Part model, mm, in its own coordinate system. Face numbers are marked on the shaded views. A direction names the side the tool comes from. Round coordinates to 2 decimals unless told otherwise and drop trailing zeros. Write each loop counter-clockwise with the first axis right and the second up, starting at its lowest first coordinate (ties: lowest second). Pieces come first, ordered by that corner, then holes.
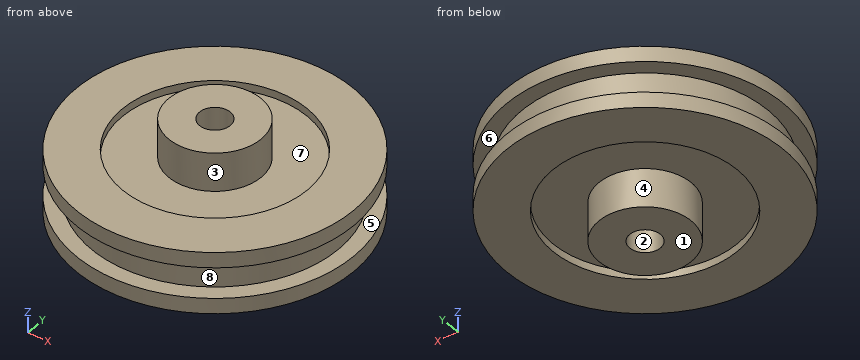
```python
from build123d import *

# Parameters (mm, degrees)
F0_R      = 9
F1_DEPTH  = 4
F2_R      = 6
F3_DEPTH  = 0.5
F4_R      = 6
F5_DEPTH  = 0.5
F6_R      = 3
F7_DEPTH  = 2.5
F8_R      = 3
F9_DEPTH  = 2.5
F10_R     = 1
F11_DEPTH = 25
F13_R     = 15.851527
F13_R_2   = 8
F14_DEPTH = 2


with BuildPart() as f1:
    # F0 (on Top) → F1 (new body)
    with BuildSketch(Plane.XY):
        Circle(F0_R)
    extrude(amount=F1_DEPTH)

    # F2 (on face) → F3 (cut)
    with BuildSketch(Plane(origin=(0, 0, 0), x_dir=(1, 0, 0), z_dir=(0, 0, -1))):
        Circle(F2_R)
    extrude(amount=-F3_DEPTH, mode=Mode.SUBTRACT)

    # F4 (on face) → F5 (cut)
    with BuildSketch(Plane.XY.offset(4)):
        Circle(F4_R)
    extrude(amount=-F5_DEPTH, mode=Mode.SUBTRACT)

    # F6 (on face) → F7 (join)
    with BuildSketch(Plane(origin=(0, 0, 0.5), x_dir=(1, 0, 0), z_dir=(0, 0, -1))):
        Circle(F6_R)
    extrude(amount=F7_DEPTH)

    # F8 (on face) → F9 (join)
    with BuildSketch(Plane.XY.offset(3.5)):
        Circle(F8_R)
    extrude(amount=F9_DEPTH)

    # F10 (on face) → F11 (cut)
    with BuildSketch(Plane.XY.offset(6)):
        Circle(F10_R)
    extrude(amount=-F11_DEPTH, mode=Mode.SUBTRACT)

    # F13 (on offset) → F14 (cut)
    with BuildSketch(Plane.XY.offset(1)):
        Circle(F13_R)
        Circle(F13_R_2, mode=Mode.SUBTRACT)
    extrude(amount=F14_DEPTH, mode=Mode.SUBTRACT)


solid = f1.part
```
Q1. Cut at D-D on y = 4.75. Write the cut outline in (x, z).
Values follow:
outline: (-7.64, 0) - (-3.67, 0) - (-3.67, 0.5) - (3.67, 0.5) - (3.67, 0) - (7.64, 0) - (7.64, 1) - (6.44, 1) - (6.44, 3) - (7.64, 3) - (7.64, 4) - (3.67, 4) - (3.67, 3.5) - (-3.67, 3.5) - (-3.67, 4) - (-7.64, 4) - (-7.64, 3) - (-6.44, 3) - (-6.44, 1) - (-7.64, 1) - close
Q2. Which spindle directions (+Z, -Z, +X, -X, +Y, -Y) get a long thin tool onto all of the face, cutting with end or side? Do the marked faces 1, 2, 3, 4 and 5. Say none if no direction does.
Values follow:
face 1: -Z, +X, -X, +Y, -Y
face 2: +Z, -Z
face 3: +Z
face 4: -Z
face 5: none
Q3. Mould opens along X. For the marked faces 6, 7 and 8 say: +X half, -X half, draft (parallel to the pull), parting line (faces both ways), or undercut.
Values follow:
face 6: draft
face 7: undercut
face 8: parting line
Q4. Cut at C-C on z = 2. Write the cut outline in (x, y), plus the area to 3 significant figures.
Values follow:
outline: circle Ø16 at (0, 0); hole circle Ø2 at (0, 0)
area: 198 mm2
Q5. Wall check: L1, parallel to Y at x = 0, z = 0.1; L2, parallel to Z at x = 0.75, y = 8.25; L3, parallel to Z at x = 3.5, y = 1.5. Give the ranges that are in metal, low to high.
Values follow:
L1: y = -9 to -6, -3 to -1, 1 to 3, 6 to 9
L2: z = 0 to 1, 3 to 4
L3: z = 0.5 to 3.5
Q6. Drop flat-ended pins along their axis: pin 1 (6 mm diameter, centred on x = 6, y = 3.5, fed in from +Z); pin 2 (2 mm diameter, centred on x = 3, z = -0.5, fed in from +Y); pin 3 (3 mm diameter, centred on x = -4.5, z = -1, fed in from +Y). Give the stop position or say it passes through.
Values follow:
pin 1: stops at z = 4
pin 2: stops at y = 8.74
pin 3: stops at y = 8.34
